Verification items for the finished model (mm, model axes). Face numbers are marked on the shaded views. Give positions to 0.01 mm unless a question says otherwise; leave off trailing zeros. Write each loop counter-clockwise with the first axis right and the second up, starting at its lowest first coordinate (ties: lowest second). Pieces come first, ordered by that corner, then holes. Notation, with made-up numbers: (44, -32.75) -> (100, -32.75) arc R14 ccw to (100, -5.75) -> close; hole circle Ø5 at (-35, 48). An arc over 180 degrees is marked (long way). Use one line per item in the form item = value. Start each with the question number.
(1) Scan lines: L1, parallel to Z at x = 0.75, y = 1.5; L2, parallel to X at y = -0.75, z = -4; L3, parallel to X at y = -1, z = -8.25. Record each from-to range of solid material in increasing order.
(2) Section check B-B, the plane z = -5. Record the cut outline in (x, y).
(3) Depth check by flat-ended pin: pin 1 Ø4 at (x, z) = (-1.5, -11) entering from +Y; pin 2 Ø1.6 at (x, y) = (0, 0) entering from +Z; pin 3 Ø2 at (x, z) = (-2, -11.5) entering from -Y. Enter the tip coordinate at first touch or a pass-through.
(4) Release check for a two-part mould opening along Y. For the marked faces 1, 2 and 3 record: pulls with the +Y half, pulls with the -Y half, needs draft (parallel to the pull), parting line crosses it, or undercut.
from build123d import *

# Parameters (mm, degrees)
SKETCH1_R           = 3.375
BOSS_EXTRUDE1_DEPTH = 1.65
SKETCH2_R           = 1.5
BOSS_EXTRUDE2_DEPTH = 14.35
CHAMFER1_SIZE       = 0.3
CUT_EXTRUDE1_DEPTH  = 2
CHAMFER2_SIZE       = 1.65


with BuildPart() as part:
    # Sketch1 → Boss-Extrude1 (new body)
    with BuildSketch(Plane.XY):
        Circle(SKETCH1_R)
    extrude(amount=BOSS_EXTRUDE1_DEPTH)

    # Sketch2 → Boss-Extrude2 (add)
    with BuildSketch(Plane(origin=(0, 0, 0), x_dir=(-1, 0, 0), z_dir=(0, 0, -1))):
        with Locations(Location((0, 0, 0), (0, 0, 180))):
            Circle(SKETCH2_R)
    extrude(amount=BOSS_EXTRUDE2_DEPTH)

    # Chamfer1
    chamfer1_edges = [part.edges().sort_by_distance(p)[0] for p in [
        (-1.5, 0, -14.35),
    ]]
    chamfer(chamfer1_edges, length=CHAMFER1_SIZE)

    # Sketch3 → Cut-Extrude1 (cut)
    with BuildSketch(Plane.XY.offset(1.65)):
        Polygon((0, 1.154700538), (-1, 0.577350269), (-1, -0.577350269), (0, -1.154700538), (1, -0.577350269), (1, 0.577350269), align=None)
    extrude(amount=-CUT_EXTRUDE1_DEPTH, mode=Mode.SUBTRACT)

    # Chamfer2
    chamfer2_edges = [part.edges().sort_by_distance(p)[0] for p in [
        (-3.375, 0, 0),
    ]]
    chamfer(chamfer2_edges, length=CHAMFER2_SIZE - 0.0001)  # a hair under: the kernel refuses the full size


solid = part.part
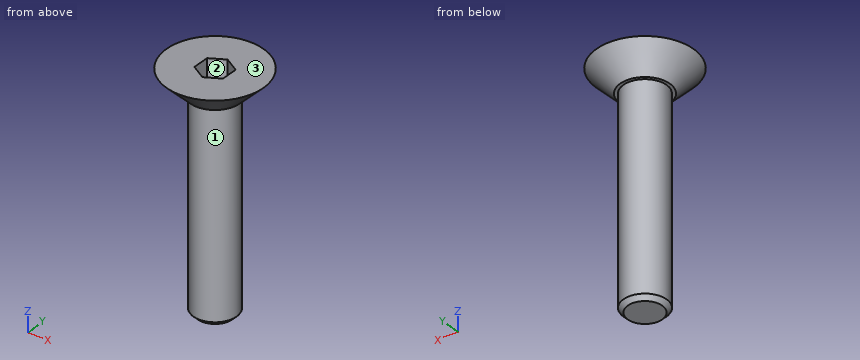
Completed:
q1.L1 = 0 to 1.65
q1.L2 = -1.3 to 1.3
q1.L3 = -1.12 to 1.12
q2.outline = circle Ø3 at (0, 0)
q3.pin_1 = 1.5
q3.pin_2 = -0.35
q3.pin_3 = -1.12
q4.face_1 = parting line crosses it
q4.face_2 = undercut
q4.face_3 = needs draft
